from build123d import *

# Parameters (mm, degrees)
SKETCH1_W           = 279.4
SKETCH1_H           = 63.5
BOSS_EXTRUDE1_DEPTH = 9.525
CUT_EXTRUDE5_DEPTH  = 10.525
CUT_EXTRUDE7_DEPTH  = 10.525
CUT_EXTRUDE8_DEPTH  = 10.525


with BuildPart() as part:
    # Sketch1 → Boss-Extrude1 (new body)
    with BuildSketch(Plane(origin=(0, 0, 0), x_dir=(1, 0, 0), z_dir=(0, 1, 0))):
        Rectangle(SKETCH1_W, SKETCH1_H)
    extrude(amount=BOSS_EXTRUDE1_DEPTH)

    # Sketch9 → Cut-Extrude5 (cut, through all)
    with BuildSketch(Plane(origin=(0, 9.525, 0), x_dir=(1, 0, 0), z_dir=(0, 1, 0))):
        with BuildLine():
            Line((-139.7, 7.969965865), (-88.9, 7.969965865))
            ThreePointArc((-88.9, 7.969965865), (-80.930034135, 0), (-88.9, -7.969965865))
            Line((-88.9, -7.969965865), (-139.7, -7.969965865))
            Line((-139.7, -7.969965865), (-139.7, 7.969965865))
        make_face()
    extrude(amount=-CUT_EXTRUDE5_DEPTH, mode=Mode.SUBTRACT)

    # Sketch12 → Cut-Extrude7 (cut, through all)
    with BuildSketch(Plane(origin=(0, 9.525, 0), x_dir=(1, 0, 0), z_dir=(0, 1, 0))):
        with BuildLine():
            Line((139.7, -8.618596636), (88.9, -8.618596636))
            ThreePointArc((88.9, -8.618596636), (80.281403364, 0), (88.9, 8.618596636))
            Line((88.9, 8.618596636), (139.7, 8.618596636))
            Line((139.7, 8.618596636), (139.7, -8.618596636))
        make_face()
    extrude(amount=-CUT_EXTRUDE7_DEPTH, mode=Mode.SUBTRACT)

    # Sketch13 → Cut-Extrude8 (cut, through all)
    with BuildSketch(Plane(origin=(0, 9.525, 0), x_dir=(1, 0, 0), z_dir=(0, 1, 0))):
        with BuildLine():
            Line((-12.7, 7.761111111), (12.7, 7.761111111))
            ThreePointArc((12.7, 7.761111111), (20.461111111, 0), (12.7, -7.761111111))
            Line((12.7, -7.761111111), (-12.7, -7.761111111))
            ThreePointArc((-12.7, -7.761111111), (-20.461111111, 0), (-12.7, 7.761111111))
        make_face()
    extrude(amount=-CUT_EXTRUDE8_DEPTH, mode=Mode.SUBTRACT)


solid = part.part
For this review, take the finished solid that the model builds, in its own axes (mm). A direction names the side the tool comes from. Give positions to 0.01 mm unless a question says otherwise; leave off trailing zeros. Order: outer loops, then holes, each group sorted by start corner. A loop starts at its lowest first (then second) coordinate and runs counter-clockwise, first axis right, second up. Notation, with made-up numbers: (-23.75, 25.5) -> (-3.75, 25.5) arc R16 ccw to (-3.75, 56.5) -> close; hole circle Ø2 at (78, 9.25). An arc over 180 degrees is marked (long way). Write item = value, one per line.
1) Draft analysis for pull direction Z (two halves, no side actions). For faces 6 (the face through (-2, 0, -15)), 7 (the face through (0, 5, 7.761)), 8 (the face through (-2, 5, -31.75)), state which applies: pulls with the +Z half, pulls with the -Z half, needs draft (parallel to the pull), parting line crosses it, or undercut.
Findings:
face_6 = needs draft
face_7 = undercut
face_8 = pulls with the -Z half
2) We need section A-A, the plane x = -99. Give the boundary of the cut face in (y, z) (3 decimals).
Findings:
outline = (0, -31.75) -> (9.525, -31.75) -> (9.525, -7.97) -> (0, -7.97) -> close; (0, 7.97) -> (9.525, 7.97) -> (9.525, 31.75) -> (0, 31.75) -> close
3) To check wall thickness, follow L1, parallel to Z at x = -96.5, y = 6; L2, parallel to Z at x = 115, y = 4.5; L3, parallel to X at y = 6, z = 3.5. State the ranges of each line that lie inside material, in increasing order. Write a range as from..to.
Findings:
L1 = -31.75..-7.97, 7.97..31.75
L2 = -31.75..-8.62, 8.62..31.75
L3 = -81.74..-19.63, 19.63..81.02
4) We need section B-B, the plane z = 0. Give the boundary of the cut face in (x, y) (3 decimals).
Findings:
outline = (-80.93, 0) -> (-20.461, 0) -> (-20.461, 9.525) -> (-80.93, 9.525) -> close; (20.461, 0) -> (80.281, 0) -> (80.281, 9.525) -> (20.461, 9.525) -> close
5) For faces 1 (the face through (139.7, 5, -20)), 2 (the face through (-114, 5, 7.97)), 3 (the face through (0, 5, -7.761)), 4 (the face through (115, 5, 8.619)), 5 (the face through (-139.7, 5, -20)), list the 3-axis set-ups (+Z, -Z, +X, -X, +Y, -Y) from which the entire face can be reached by the end or side of a thin tool; tool diameter is ignored.
Findings:
face_1 = +Z, -Z, +X, +Y, -Y
face_2 = -X, +Y, -Y
face_3 = +Y, -Y
face_4 = +X, +Y, -Y
face_5 = +Z, -Z, -X, +Y, -Y
6) We need section C-C, the plane y = 3. Give the boundary of the cut face in (x, z).
Findings:
outline = (-139.7, -31.75) -> (139.7, -31.75) -> (139.7, -8.62) -> (88.9, -8.62) arc R8.62 cw to (88.9, 8.62) -> (139.7, 8.62) -> (139.7, 31.75) -> (-139.7, 31.75) -> (-139.7, 7.97) -> (-88.9, 7.97) arc R7.97 cw to (-88.9, -7.97) -> (-139.7, -7.97) -> close; hole (-12.7, -7.76) -> (12.7, -7.76) arc R7.76 ccw to (12.7, 7.76) -> (-12.7, 7.76) arc R7.76 ccw to start
7) Insertion check: pin 1 (3 mm diameter, centred on y = 5.5, z = -8.5, fed in from +X). The pin has a flat end and moves straight along its axis. Give the tip position at first contact, or say it passes through.
Findings:
pin_1 = 139.7
